Source: CAD feature listing. Evaluate the final solid. Frame: model axes, mm. A direction names the side the tool comes from. Give positions to 0.01 mm unless a question says otherwise; leave off trailing zeros. Loops run counter-clockwise (first coordinate to the right, second up) from the corner with the lowest first, then second, coordinate; pieces in that order, holes last. Notation, with made-up numbers: (-34.75, 85.5) -> (21.25, 85.5) arc R36 cw to (21.25, 121.5) -> close; hole circle Ø7 at (-23, -19). An arc over 180 degrees is marked (long way). Answer as a JSON object with one key per item and string values. Group by question number.
from build123d import *

# Parameters (mm, degrees)
ESQUISSE1_R      = 40
ESQUISSE1_R_2    = 38
EXTRUSION1_DEPTH = 40
EXTRUSION2_DEPTH = 5


with BuildPart() as part:
    # Esquisse1 → Extrusion1 (new body)
    with BuildSketch(Plane(origin=(0, 0, 0), x_dir=(1, 0, 0), z_dir=(0, 1, 0))):
        Circle(ESQUISSE1_R)
        Circle(ESQUISSE1_R_2, mode=Mode.SUBTRACT)
    extrude(amount=EXTRUSION1_DEPTH)

    # Esquisse2 → Extrusion2 (cut)
    with BuildSketch(Plane(origin=(0, 40, 0), x_dir=(1, 0, 0), z_dir=(0, 1, 0))):
        with BuildLine():
            Line((0, -40), (0, -38))
            ThreePointArc((0, -38), (-1.000346681, -37.986830699), (-2, -37.947331922))
            Line((-2, -37.947331922), (-2.105263158, -39.944559918))
            ThreePointArc((-2.105263158, -39.944559918), (-1.052996506, -39.986137577), (0, -40))
        make_face()
        with BuildLine():
            Line((0, 40), (0, 38))
            ThreePointArc((0, 38), (1.000346681, 37.986830699), (2, 37.947331922))
            Line((2, 37.947331922), (2.105263158, 39.944559918))
            ThreePointArc((2.105263158, 39.944559918), (1.052996506, 39.986137577), (0, 40))
        make_face()
        with BuildLine():
            Line((22.096109748, 33.343094247), (20.991304261, 31.675939535))
            ThreePointArc((20.991304261, 31.675939535), (21.817611901, 31.112566769), (22.628807775, 30.527644172))
            Line((22.628807775, 30.527644172), (23.819797658, 32.134362286))
            ThreePointArc((23.819797658, 32.134362286), (22.965907264, 32.750070283), (22.096109748, 33.343094247))
        make_face()
        with BuildLine():
            Line((-20.311213778, -34.459463067), (-19.295653089, -32.736489913))
            ThreePointArc((-19.295653089, -32.736489913), (-20.150457189, -32.217372256), (-20.991304261, -31.675939535))
            Line((-20.991304261, -31.675939535), (-22.096109748, -33.343094247))
            ThreePointArc((-22.096109748, -33.343094247), (-21.211007567, -33.913023427), (-20.311213778, -34.459463067))
        make_face()
    extrude(amount=-EXTRUSION2_DEPTH, mode=Mode.SUBTRACT)


solid = part.part
(1) First-contact query: pin 1 (8 mm diameter, centred on y = 17, z = -28, fed in from +X); pin 2 (6 mm diameter, centred on x = 8.5, y = 10.5, fed in from -Z); pin 3 (4 mm diameter, centred on y = 15, z = -10, fed in from +X). Flat tips, straight axial feed; report the tip coordinate or a pass-through.
(2) Section query A-A on z = 0. Return the cut outline in (x, y), plus the area to 3 significant figures.
(3) Mould query, pull axis X, two halves, no side actions, for faces 5 (the face through (-11, 40, 37)), 6 (the face through (-1, 35, 39)), 7 (the face through (-8.67, 19.72, 39.05)), 8 (the face through (-21, 35, 33)). Classes: pulls with the +X half, pulls with the -X half, needs draft (parallel to the pull), parting line crosses it, or undercut.
(4) Section query C-C on y = 13.5. Return the cut outline in (x, z), plus the area to 3 significant figures.
(5) Section query B-B on x = 4. Return the cut outline in (y, z), plus the area to 3 significant figures.
(6) Material intervals for line 1 (Z direction, x = 0, y = 25); line 2 (X direction, y = 12, z = 25), sorted ascending. Write a range as from..to.
(7) Access query for faces 1 (the face through (36, 40, 14)), 2 (the face through (-2.05, 37.53, 38.93)), 3 (the face through (2.05, 37.53, -38.93)), 4 (the face through (22, 35, -32)). Directions: +Z, -Z, +X, -X, +Y, -Y. A direction counts if a zero-diameter tool reaches every point of the face in a straight line with its end or side. Return the directions, or none.
Result:
{
 "1": {"pin 1": "x = 32", "pin 2": "z = -39.62", "pin 3": "x = 39.19"},
 "2": {"outline": "(-40, 0) -> (-38, 0) -> (-38, 40) -> (-40, 40) -> close; (38, 0) -> (40, 0) -> (40, 40) -> (38, 40) -> close", "area": "160 mm²"},
 "3": {"face 5": "needs draft", "face 6": "undercut", "face 7": "parting line crosses it", "face 8": "undercut"},
 "4": {"outline": "circle Ø80 at (0, 0); hole circle Ø76 at (0, 0)", "area": "490 mm²"},
 "5": {"outline": "(0, -39.8) -> (40, -39.8) -> (40, -37.79) -> (0, -37.79) -> close; (0, 37.79) -> (40, 37.79) -> (40, 39.8) -> (0, 39.8) -> close", "area": "161 mm²"},
 "6": {"line 1": "-40..-38, 38..40", "line 2": "-31.22..-28.62, 28.62..31.22"},
 "7": {"face 1": "+Z, -Z, +X, -X, +Y", "face 2": "+Z, +Y", "face 3": "-Z, +Y", "face 4": "+Y"}
}
